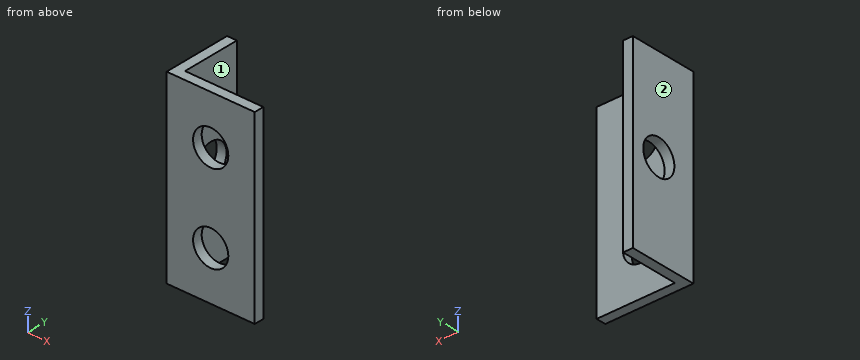
from build123d import *

# Parameters (mm, degrees)
F1_DEPTH = 95
F2_R     = 9
F3_DEPTH = 25
F4_R     = 9
F5_DEPTH = 25


with BuildPart() as f1:
    # F0 (on Top) → F1 (new body)
    with BuildSketch(Plane.XY):
        Polygon((0, 0), (0, 30), (-5, 30), (-5, -5), (40, -5), (40, 0), align=None)
    extrude(amount=F1_DEPTH)

    # F2 (on face) → F3 (cut)
    with BuildSketch(Plane.XZ.offset(5)):
        with Locations((17.5, 70)):
            Circle(F2_R)
        with Locations((17.5, 25)):
            Circle(F2_R)
    extrude(amount=-F3_DEPTH, mode=Mode.SUBTRACT)

    # F4 (on face) → F5 (cut)
    with BuildSketch(Plane.YZ):
        with Locations((15, 47.5)):
            Circle(F4_R)
    extrude(amount=-F5_DEPTH, mode=Mode.SUBTRACT)


solid = f1.part
Part model, mm, in its own coordinate system. Face numbers are marked on the shaded views. A direction names the side the tool comes from. Give positions to 0.01 mm unless a question says otherwise; leave off trailing zeros. Write each loop counter-clockwise with the first axis right and the second up, starting at its lowest first coordinate (ties: lowest second). Pieces come first, ordered by that corner, then holes.
1) Probe L1, parallel to Z at x = 17, y = -1; L2, parallel to Y at x = -2, z = 47; L3, parallel to Z at x = -3.2, y = 15. List the from-to ranges inside material, lowest first.
Resolved:
L1: z = 0 to 16.01, 33.99 to 61.01, 78.99 to 95
L2: y = -5 to 6.01, 23.99 to 30
L3: z = 0 to 38.5, 56.5 to 95
2) Cut at A-A on z = 47.5. Write the cut outline in (x, y), then the cut area to 3 significant figures.
Resolved:
outline: (-5, -5) - (40, -5) - (40, 0) - (0, 0) - (0, 6) - (-5, 6) - close; (-5, 24) - (0, 24) - (0, 30) - (-5, 30) - close
area: 285 mm2
3) Cut at B-B on y = 15. Write the cut outline in (x, z).
Resolved:
outline: (-5, 0) - (0, 0) - (0, 38.5) - (-5, 38.5) - close; (-5, 56.5) - (0, 56.5) - (0, 95) - (-5, 95) - close
4) Cut at C-C on x = 17.5. Write the cut outline in (y, z), then the cut area to 3 significant figures.
Resolved:
outline: (-5, 0) - (0, 0) - (0, 16) - (-5, 16) - close; (-5, 34) - (0, 34) - (0, 61) - (-5, 61) - close; (-5, 79) - (0, 79) - (0, 95) - (-5, 95) - close
area: 295 mm2
5) Cut at D-D on z = 14.5. Write the cut outline in (x, y), then the cut area to 3 significant figures.
Resolved:
outline: (-5, -5) - (40, -5) - (40, 0) - (0, 0) - (0, 30) - (-5, 30) - close
area: 375 mm2
6) Pin check, flat tips, straight feed: pin 1 (6 mm diameter, centred on x = 8, y = 5, fed in from +Z); pin 2 (12 mm diameter, centred on x = 32, z = 47.5, fed in from +Y); pin 3 (9 mm diameter, centred on y = 14.5, z = 65, fed in from +X). Stop position of each tip, or through.
Resolved:
pin 1: passes through
pin 2: stops at y = 0
pin 3: stops at x = 0
7) Which spindle directions (+Z, -Z, +X, -X, +Y, -Y) get a long thin tool onto all of the face, cutting with end or side? Do the marked faces 1 and 2. Say none if no direction does.
Resolved:
face 1: +Z, -Z, +X, +Y
face 2: +Z, -Z, -X, +Y, -Y
